```python
from build123d import *

# Parameters (mm, degrees)
F1_DEPTH = 3


with BuildPart() as f1:
    # F0 (on Front) → F1 (new body)
    with BuildSketch(Plane.XZ):
        Polygon((-75, 50), (-95, 70), (-95, -70), (-75, -50), align=None)
        Polygon((95, 70), (-95, 70), (-75, 50), (75, 50), align=None)
        Polygon((95, -70), (95, 70), (75, 50), (75, -50), align=None)
        Polygon((-75, -50), (-95, -70), (95, -70), (75, -50), align=None)
    extrude(amount=F1_DEPTH)


solid = f1.part
```
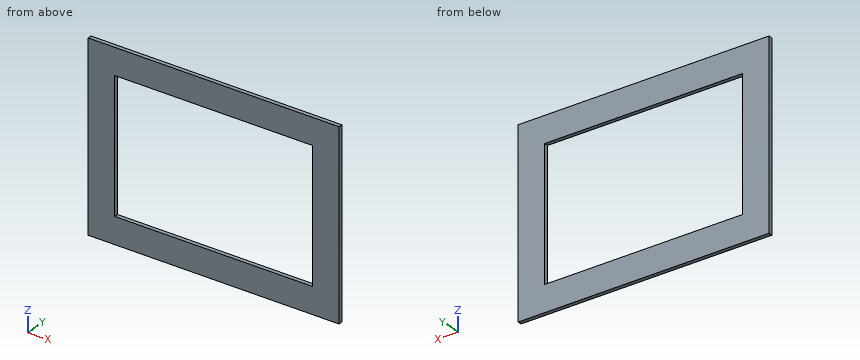
Geometry check sheet. Reference: the model listing, model coordinates, mm. Round coordinates to 2 decimals unless told otherwise and drop trailing zeros. Write each loop counter-clockwise with the first axis right and the second up, starting at its lowest first coordinate (ties: lowest second). Pieces come first, ordered by that corner, then holes. Notation, with made-up numbers: (68, -10.75) - (125, -10.75) arc R18 cw to (125, 3.25) - close; hole circle Ø3 at (62.5, -38.5). An arc over 180 degrees is marked (long way). Write each question's results on one line, items separated by ' | '.
(1) Thickness scan on probe 1 along Z at (x, y) = (-31.5, -1.75); probe 2 along X at (y, z) = (-0.85, 30). Record the ranges inside material, lowest first. Write a range as from..to.
Computed:
probe 1: z = -70..-50, 50..70 | probe 2: x = -95..-75, 75..95
(2) Sectioned sample at A-A, the plane z = -8.5. Enter the section's corners in (x, y), plus the area to 3 significant figures.
Computed:
outline: (-95, -3) - (-75, -3) - (-75, 0) - (-95, 0) - close; (75, -3) - (95, -3) - (95, 0) - (75, 0) - close | area: 120 mm^2
(3) Sectioned sample at C-C, the plane y = -2. Enter the section's corners in (x, z), plus the area to 3 significant figures.
Computed:
outline: (-95, -70) - (95, -70) - (95, 70) - (-95, 70) - close; hole (-75, -50) - (75, -50) - (75, 50) - (-75, 50) - close | area: 11,600 mm^2
(4) Sectioned sample at B-B, the plane x = -56. Enter the section's corners in (y, z).
Computed:
outline: (-3, -70) - (0, -70) - (0, -50) - (-3, -50) - close; (-3, 50) - (0, 50) - (0, 70) - (-3, 70) - close
